from build123d import *

# Parameters (mm, degrees)
BOX014_W           = 67
BOX014_H           = 180
BOX014_DEPTH       = 116
BOX014_PITCH_ANGLE = 12.5
BOX012_W           = 66.5
BOX012_H           = 180
BOX012_DEPTH       = 116
BOX015_W           = 67
BOX015_H           = 180
BOX015_DEPTH       = 116
BOX015_PITCH_ANGLE = 12.5
BOX013_W           = 67.5
BOX013_H           = 180
BOX013_DEPTH       = 117


with BuildPart() as cube415:
    # Box014 → Box014 (new body)
    with BuildSketch(Plane.XY):
        with Locations((33.5, 90)):
            Rectangle(BOX014_W, BOX014_H)
    extrude(amount=BOX014_DEPTH)


with BuildPart() as cube415_1:
    # Box014 pitch: moved
    add(cube415.part.rotate(Axis((0, 0, 0), (0, 1, 0)), BOX014_PITCH_ANGLE))


with BuildPart() as cube415_2:
    # Box014 placement: moved
    add(cube415_1.part.moved(Location((-53.2, 0, 65))))


with BuildPart() as cut333:
    # Box012 → Box012 (new body)
    with BuildSketch(Plane(origin=(14.5, 0, -0.5), x_dir=(1, 0, 0), z_dir=(0, 0, 1))):
        with Locations((33.25, 90)):
            Rectangle(BOX012_W, BOX012_H)
    extrude(amount=BOX012_DEPTH)

    # Cut006: cut Cube415
    add(cube415_2.part, mode=Mode.SUBTRACT)


with BuildPart() as cut333_1:
    # Cut006 placement: moved
    add(cut333.part.moved(Location((0, -2, 0))))


with BuildPart() as cube417:
    # Box015 → Box015 (new body)
    with BuildSketch(Plane.XY):
        with Locations((33.5, 90)):
            Rectangle(BOX015_W, BOX015_H)
    extrude(amount=BOX015_DEPTH)


with BuildPart() as cube417_1:
    # Box015 pitch: moved
    add(cube417.part.rotate(Axis((0, 0, 0), (0, 1, 0)), BOX015_PITCH_ANGLE))


with BuildPart() as cube417_2:
    # Box015 placement: moved
    add(cube417_1.part.moved(Location((-53.7, 0, 65))))


with BuildPart() as cut008:
    # Box013 → Box013 (new body)
    with BuildSketch(Plane(origin=(14, 0, -1), x_dir=(1, 0, 0), z_dir=(0, 0, 1))):
        with Locations((33.75, 90)):
            Rectangle(BOX013_W, BOX013_H)
    extrude(amount=BOX013_DEPTH)

    # Cut005: cut Cube417
    add(cube417_2.part, mode=Mode.SUBTRACT)


with BuildPart() as cut008_1:
    # Cut005 placement: moved
    add(cut008.part.moved(Location((0, -2, 0))))

    # Cut008: cut Cut333
    add(cut333_1.part, mode=Mode.SUBTRACT)


with BuildPart() as cut008_2:
    # Cut008 placement: moved
    add(cut008_1.part.moved(Location((0.5, -3, 0.5))))


solid = cut008_2.part
Input: part model. Units: mm. Frame: model coordinates. A direction names the side the tool comes from. Round coordinates to 2 decimals unless told otherwise and drop trailing zeros. Order: outer loops, then holes, each group sorted by start corner. A loop starts at its lowest first (then second) coordinate and runs counter-clockwise, first axis right, second up.
1. Pin query (flat end, axial travel): P1, Ø2, axis at y = 135.5, z = 90, coming from the -X side; P2, Ø10, axis at y = 112, z = 73.5, coming from the -X side. Return the tip coordinate at first contact, or that it passes through.
The answers:
P1: stops at x = 20.64
P2: stops at x = 16.09
2. Set-up query: faces 1 (the face through (48, 86, 0)), 2 (the face through (54, 86, 116.5)). Return all of +Z, -Z, +X, -X, +Y, -Y with unobstructed straight access to the full face (end or side cutting, diameter ignored); none if empty.
The answers:
face 1: +Y, -Y
face 2: +Z, +X, -X, +Y, -Y
3. Mould query, pull axis X, two halves, no side actions, for faces 3 (the face through (82, 84, 57)), 4 (the face through (15, 84, 30)), 5 (the face through (20.53, 83.74, 88.52)). Classes: released by +X, released by -X, zero draft, split by the parting line, or undercut.
The answers:
face 3: released by +X
face 4: undercut
face 5: released by -X
4. Material intervals for line 1 (X direction, y = 66.5, z = 42); line 2 (Z direction, x = 31, y = 53.5); line 3 (X direction, y = 7.5, z = 72), sorted ascending.
The answers:
line 1: x = 14.5 to 15, 81.5 to 82
line 2: z = -0.5 to 0, 116 to 116.5
line 3: x = 16.87 to 17.37, 81.5 to 82
5. Cut plane B-B, the plane y = 17. Output: boundary loops of the cut face in (x, z), then the cut area to 3 significant figures.
The answers:
outline: (14.5, -0.5) - (82, -0.5) - (82, 116.5) - (26.73, 116.5) - (14.5, 61.32) - close; hole (15, 0) - (81.5, 0) - (81.5, 116) - (27.12, 116) - (15, 61.32) - close
area: 177 mm2
6. Cut plane A-A, the plane x = 47.5. Output: boundary loops of the cut face in (y, z), then the cut area to 3 significant figures.
The answers:
outline: (-5, -0.5) - (175, -0.5) - (175, 0) - (-5, 0) - close; (-5, 116) - (175, 116) - (175, 116.5) - (-5, 116.5) - close
area: 180 mm2
7. Cut plane C-C, the plane z = 79. Output: boundary loops of the cut face in (x, y), then the cut area to 3 significant figures.
The answers:
outline: (18.42, -5) - (18.92, -5) - (18.92, 175) - (18.42, 175) - close; (81.5, -5) - (82, -5) - (82, 175) - (81.5, 175) - close
area: 180 mm2
